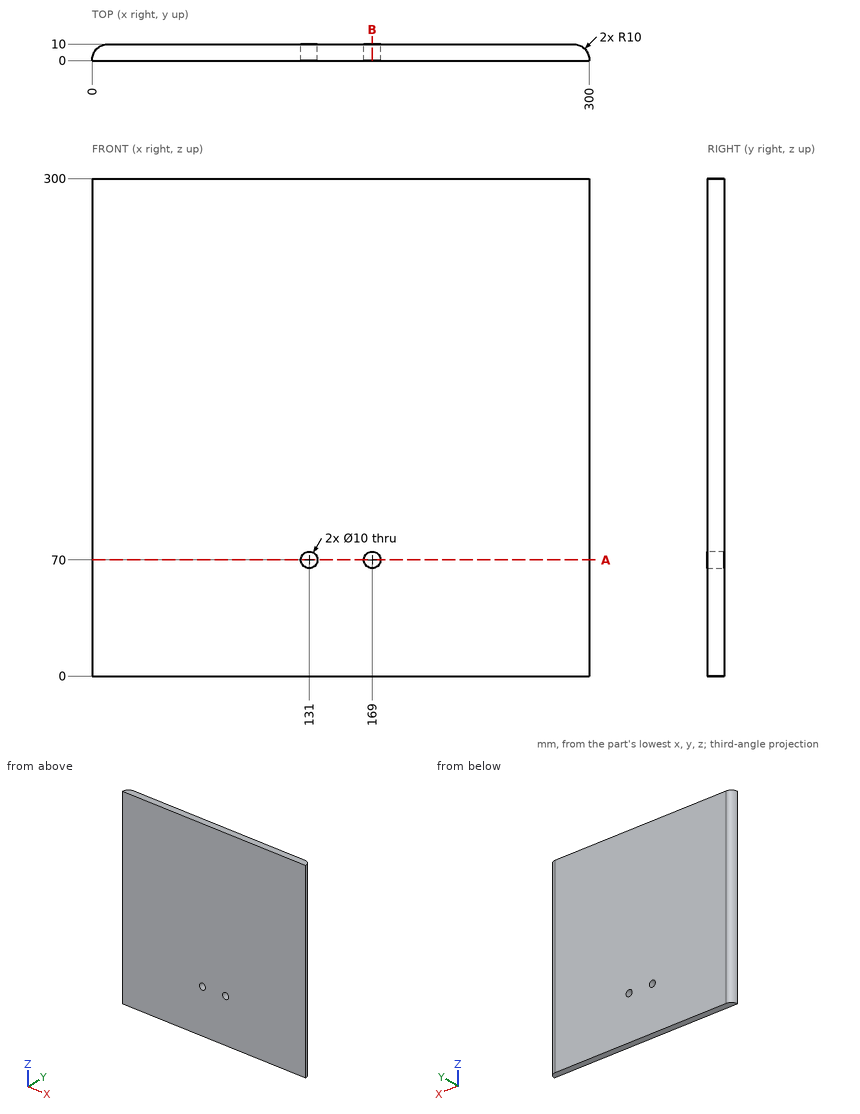
Input: dimensioned drawing with shaded views. Units: mm. Origin: part minimum x, y, z. Give positions to 0.01 mm unless a question says otherwise; leave off trailing zeros. Write each loop counter-clockwise with the first axis right and the second up, starting at its lowest first coordinate (ties: lowest second). Pieces come first, ordered by that corner, then holes. Notation, with made-up numbers: (47, -1) -> (103, -1) arc R8 ccw to (103, 12) -> close; hole circle Ø8 at (-7.75, 21.25). An arc over 180 degrees is marked (long way). Answer as a JSON object with one key per item and string values.
1. Cut plane B-B on x = 169. Output: boundary loops of the cut face in (y, z).
Ans:
{"outline": "(0, 0) -> (10, 0) -> (10, 65) -> (0, 65) -> close; (0, 75) -> (10, 75) -> (10, 300) -> (0, 300) -> close"}
2. Ray query, probe 1 along X at (y, z) = (2, 70); probe 2 along X at (y, z) = (6.75, 70); probe 3 along Z at (x, y) = (129, 7). Return the intervals inside material, ascending. Write a range as from..to.
Ans:
{"probe 1": "x = 0.2..126, 136..164, 174..299.8", "probe 2": "x = 2.62..126, 136..164, 174..297.38", "probe 3": "z = 0..65.42, 74.58..300"}
3. Contact query for flat-ended pins moving along their axis: pin 1 (4 mm diameter, centred on y = 4, z = 154, fed in from -X); pin 2 (8 mm diameter, centred on x = 131, z = 70, fed in from -Y); pin 3 (5 mm diameter, centred on y = 8, z = 160.5, fed in from -X). Output: stop coordinate, or through.
Ans:
{"pin 1": "stops at x = 0.2", "pin 2": "passes through", "pin 3": "stops at x = 1.65"}
4. Cut plane A-A on z = 70. Count the separate pieces of the cut face and the enclosed holes in it, and give its area (3 significant figures).
Ans:
{"separate pieces": "3", "enclosed holes": "0", "area": "2,760 mm^2"}
